```python
from build123d import *

# Parameters (mm, degrees)
SKETCH1_R           = 1.125
SKETCH1_R_2         = 2.5
SKETCH1_R_3         = 3.5
BOSS_EXTRUDE1_DEPTH = 2
SKETCH2_R           = 4
BOSS_EXTRUDE2_DEPTH = 2
SKETCH3_R           = 1.75
CUT_EXTRUDE1_DEPTH  = 5
SKETCH4_R           = 3.25
SKETCH4_R_2         = 1.75
CUT_EXTRUDE2_DEPTH  = 2
SKETCH6_W           = 20
SKETCH6_H           = 2.75
BOSS_EXTRUDE3_DEPTH = 4
CUT_EXTRUDE3_DEPTH  = 16
FILLET1_R           = 2
FILLET2_R           = 1


with BuildPart() as part:
    # Sketch1 → Boss-Extrude1 (new body)
    with BuildSketch(Plane(origin=(0, 0, 0), x_dir=(1, 0, 0), z_dir=(0, 1, 0))):
        with BuildLine():
            Line((25, -31), (-25, -31))
            ThreePointArc((-25, -31), (-28.535533906, -29.535533906), (-30, -26))
            Line((-30, -26), (-30, 26))
            ThreePointArc((-30, 26), (-28.535533906, 29.535533906), (-25, 31))
            Line((-25, 31), (25, 31))
            ThreePointArc((25, 31), (28.535533906, 29.535533906), (30, 26))
            Line((30, 26), (30, -26))
            ThreePointArc((30, -26), (28.535533906, -29.535533906), (25, -31))
        make_face()
        with Locations((-13.5, -23.25)):
            Circle(SKETCH1_R, mode=Mode.SUBTRACT)
        with Locations((-4, -23.25)):
            Circle(SKETCH1_R, mode=Mode.SUBTRACT)
        with Locations((14.5, -23.25)):
            Circle(SKETCH1_R_2, mode=Mode.SUBTRACT)
        with Locations((5, -23.25)):
            Circle(SKETCH1_R_3, mode=Mode.SUBTRACT)
    extrude(amount=BOSS_EXTRUDE1_DEPTH)

    # Sketch2 → Boss-Extrude2 (add)
    with BuildSketch(Plane.XZ):
        with Locations((-22.25, 23.25)):
            Circle(SKETCH2_R)
        with Locations((22.25, 23.25)):
            Circle(SKETCH2_R)
    extrude(amount=BOSS_EXTRUDE2_DEPTH)

    # Sketch3 → Cut-Extrude1 (cut, through all)
    with BuildSketch(Plane.XZ.offset(2)):
        with Locations((-22.25, 23.25)):
            Circle(SKETCH3_R)
        with Locations((22.25, 23.25)):
            Circle(SKETCH3_R)
    extrude(amount=-CUT_EXTRUDE1_DEPTH, mode=Mode.SUBTRACT)

    # Sketch4 → Cut-Extrude2 (cut)
    with BuildSketch(Plane(origin=(0, 2, 0), x_dir=(1, 0, 0), z_dir=(0, 1, 0))):
        with Locations((-22.25, -23.25)):
            Circle(SKETCH4_R)
        with Locations((-22.25, -23.25)):
            Circle(SKETCH4_R_2, mode=Mode.SUBTRACT)
        with Locations((22.25, -23.25)):
            Circle(SKETCH4_R)
        with Locations((22.25, -23.25)):
            Circle(SKETCH4_R_2, mode=Mode.SUBTRACT)
    extrude(amount=-CUT_EXTRUDE2_DEPTH, mode=Mode.SUBTRACT)

    # Sketch6 → Boss-Extrude3 (add)
    with BuildSketch(Plane.XZ):
        with Locations((0, -27.625)):
            Rectangle(SKETCH6_W, SKETCH6_H)
    extrude(amount=BOSS_EXTRUDE3_DEPTH)

    # Sketch7 → Cut-Extrude3 (cut)
    with BuildSketch(Plane(origin=(8, 0, 0), x_dir=(0, 0, -1), z_dir=(1, 0, 0))):
        Polygon((29, -3), (27, 0), (29, 0), align=None)
    extrude(amount=-CUT_EXTRUDE3_DEPTH, mode=Mode.SUBTRACT)

    # Fillet1
    fillet1_edges = [part.edges().sort_by_distance(p)[0] for p in [
        (10, -4, -27.625),
        (-10, -4, -27.625),
    ]]
    fillet(fillet1_edges, radius=FILLET1_R)

    # Fillet2
    fillet2_edges = [part.edges().sort_by_distance(p)[0] for p in [
        (28.535533906, 2, -29.535533906),
        (0, 2, -31),
        (-28.535533906, 2, -29.535533906),
        (-30, 2, 0),
        (-28.535533906, 2, 29.535533906),
        (0, 2, 31),
        (28.535533906, 2, 29.535533906),
        (30, 2, 0),
    ]]
    fillet(fillet2_edges, radius=FILLET2_R)


solid = part.part
```
Verification items for the finished model (mm, model axes). A direction names the side the tool comes from. Give positions to 0.01 mm unless a question says otherwise; leave off trailing zeros. Order: outer loops, then holes, each group sorted by start corner. A loop starts at its lowest first (then second) coordinate and runs counter-clockwise, first axis right, second up. Notation, with made-up numbers: (-12.5, 51) -> (-0.5, 51) arc R21 ccw to (-0.5, 55) -> close; hole circle Ø11 at (-25, 37.25). An arc over 180 degrees is marked (long way). Use a Markdown table: item, result.
1) Section check D-D, the plane z = -5. Record the boundary of the cut face in (x, y), then the cut area to 3 significant figures.
Results:
| item | result |
|---|---|
| outline | (-30, 0) -> (30, 0) -> (30, 1) arc R1 ccw to (29, 2) -> (-29, 2) arc R1 ccw to (-30, 1) -> close |
| area | 120 mm² |
2) Section check A-A, the plane x = -13.5. Record the boundary of the cut face in (y, z) (3 decimals).
Results:
| item | result |
|---|---|
| outline | (0, -31) -> (1, -31) arc R1 ccw to (2, -30) -> (2, 22.125) -> (0, 22.125) -> close; (0, 24.375) -> (2, 24.375) -> (2, 30) arc R1 ccw to (1, 31) -> (0, 31) -> close |
3) Section check C-C, the plane x = -22.25. Record the boundary of the cut face in (y, z).
Results:
| item | result |
|---|---|
| outline | (-2, 19.25) -> (0, 19.25) -> (0, -31) -> (1, -31) arc R1 ccw to (2, -30) -> (2, 20) -> (0, 20) -> (0, 21.5) -> (-2, 21.5) -> close; (-2, 25) -> (0, 25) -> (0, 26.5) -> (2, 26.5) -> (2, 30) arc R1 ccw to (1, 31) -> (0, 31) -> (0, 27.25) -> (-2, 27.25) -> close |
4) Mould release check, pull along X, two halves, no side actions. Record for faces 1 (the flat face through (0, 2, 0)), 2 (the cylindrical face through (-28.57, 0.49, -29.5)), 3 (the cylindrical face through (-23.54, -1.01, 24.43)): pulls with the +X half, pulls with the -X half, needs draft (parallel to the pull), parting line crosses it, or undercut.
Results:
| item | result |
|---|---|
| face 1 | needs draft |
| face 2 | pulls with the -X half |
| face 3 | undercut |
5) Tool access check on faces 4 (the flat face through (24, 0, 25)), 5 (the flat face through (10, -1, -28)), 6 (the cylindrical face through (19.3, -0.99, 25.95)). Record the directions out of +Z, -Z, +X, -X, +Y, -Y that give a thin tool (end or side, any length) a straight path to the whole face; none if there is none.
Results:
| item | result |
|---|---|
| face 4 | +Y |
| face 5 | +Z, -Z, +X, -Y |
| face 6 | -Y |
6) Material ranges on probe 1 along Z at (x, y) = (14.5, 0.45); probe 2 along Z at (x, y) = (22.25, 0.6); probe 3 along Y at (x, z) = (-17.5, -20), recorded low to high.
Results:
| item | result |
|---|---|
| probe 1 | -31 to 20.75, 25.75 to 31 |
| probe 2 | -31 to 20, 26.5 to 31 |
| probe 3 | 0 to 2 |
7) Depth check by flat-ended pin: pin 1 Ø0.6 at (y, z) = (-0.5, -28) entering from +X; pin 2 Ø2 at (y, z) = (-1.5, -28) entering from -X; pin 3 Ø6 at (x, z) = (22.25, 23.25) entering from +Y. Enter the tip coordinate at first touch or a pass-through.
Results:
| item | result |
|---|---|
| pin 1 | x = 10 |
| pin 2 | x = -10 |
| pin 3 | y = 0 |
8) Section check B-B, the plane y = -0.8. Record the boundary of the cut face in (x, z).
Results:
| item | result |
|---|---|
| outline | circle Ø8 at (-22.25, 23.25); (-10, -29) -> (-8, -29) -> (-8, -27.53) -> (8, -27.53) -> (8, -29) -> (10, -29) -> (10, -26.25) -> (-10, -26.25) -> close; circle Ø8 at (22.25, 23.25); hole circle Ø3.5 at (-22.25, 23.25); hole circle Ø3.5 at (22.25, 23.25) |
